```python
from build123d import *

# Parameters (mm, degrees)
F0_W     = 84
F0_H     = 80
F0_R     = 14
F0_R_2   = 16
F1_DEPTH = 225
F2_R     = 16
F2_R_2   = 14
F3_DEPTH = 100
F4_SIZE  = 1
F5_R     = 2.5
F6_DEPTH = 25
F7_R     = 2.5
F8_DEPTH = 25


# Not quite as in the source:
# - a feature names something its author has since deleted; it is built from what else it names


with BuildPart() as f1:
    # F0 (on Front) → F1 (new body)
    with BuildSketch(Plane.XZ):
        Rectangle(F0_W, F0_H)
        with Locations((-21, -19)):
            Circle(F0_R, mode=Mode.SUBTRACT)
        with Locations((21, -19)):
            Circle(F0_R_2, mode=Mode.SUBTRACT)
    extrude(amount=-F1_DEPTH)

    # F2 (on face) → F3 (cut)
    with BuildSketch(Plane(origin=(-42, 0, 0), x_dir=(0, -1, 0), z_dir=(-1, 0, 0))):
        with Locations((-204, 19)):
            Circle(F2_R)
        with Locations((-56, 19)):
            Circle(F2_R_2)
        with Locations((-21, 19)):
            Circle(F2_R)
    extrude(amount=-F3_DEPTH, mode=Mode.SUBTRACT)

    # F4
    f4_edges = [f1.edges().sort_by_distance(p)[0] for p in [
        (-42, 220, 19),
        (-42, 70, 19),
        (-42, 37, 19),
        (-35, 0, -19),
        (5, 0, -19),
        (42, 37, 19),
        (42, 70, 19),
        (42, 220, 19),
    ]]
    chamfer(f4_edges, length=F4_SIZE)

    # F5 (on face) → F6 (cut)
    with BuildSketch(Plane.XY.offset(40)):
        with Locations((21, 204)):
            Circle(F5_R)
        with Locations((21, 56)):
            Circle(F5_R)
        with Locations((21, 21)):
            Circle(F5_R)
        with Locations((-21, 21)):
            Circle(F5_R)
        with Locations((-21, 56)):
            Circle(F5_R)
        with Locations((-21, 204)):
            Circle(F5_R)
    extrude(amount=-F6_DEPTH, mode=Mode.SUBTRACT)

    # F7 (on face) → F8 (cut)
    with BuildSketch(Plane(origin=(0, 0, -40), x_dir=(1, 0, 0), z_dir=(0, 0, -1))):
        with Locations((-21, -21)):
            Circle(F7_R)
        with Locations((21, -21)):
            Circle(F7_R)
        with BuildLine():
            ThreePointArc((-18.5, -105), (-22.767766953, -103.232233047), (-21, -107.5))
            ThreePointArc((-21, -107.5), (-19.232233047, -106.767766953), (-18.5, -105))
        make_face()
        with BuildLine():
            ThreePointArc((-21, -152.5), (-22.767766953, -156.767766953), (-18.5, -155))
            ThreePointArc((-18.5, -155), (-19.232233047, -153.232233047), (-21, -152.5))
        make_face()
        with Locations((-21, -204)):
            Circle(F7_R)
        with Locations((21, -204)):
            Circle(F7_R)
    extrude(amount=-F8_DEPTH, mode=Mode.SUBTRACT)


solid = f1.part
```
Input: part model. Units: mm. Frame: model coordinates. A direction names the side the tool comes from. Coordinates: 2 decimals unless noted, no trailing zeros. Write each loop counter-clockwise with the first axis right and the second up, starting at its lowest first coordinate (ties: lowest second). Pieces come first, ordered by that corner, then holes.
1) Material intervals for line 1 along X through (y, z) = (56, 36); line 2 along Y through (x, z) = (-21, 38); line 3 along Y through (x, z) = (-21, -37), sorted ascending.
2) Mould query, pull axis Z, two halves, no side actions, for faces 1 (the flat face through (-1, 111, 40)), 2 (the cylindrical face through (-0.57, 24.47, 3.38)), 3 (the cylindrical face through (-0.574, 43.068, 13.638)), 4 (the cylindrical face through (-23.5, 20.9, -36.4)). Classes: pulls with the +Z half, pulls with the -Z half, needs draft (parallel to the pull), parting line crosses it, or undercut.
3) Section B-B on z = -19. Output: boundary loops of the cut face in (x, y), and give its area (3 significant figures).
4) Set-up query: faces 5 (the cylindrical face through (20.67, 206.48, 37.44)), 6 (the cylindrical face through (17.53, 111.43, -34.62)), 7 (the cylindrical face through (20.67, 201.52, -37.44)). Return all of +Z, -Z, +X, -X, +Y, -Y with unobstructed straight access to the full face (end or side cutting, diameter ignored); none if empty.
5) Section C-C on y = 204. Output: boundary loops of the cut face in (x, z).
6) Pin query (flat end, axial travel): pin 1 Ø3 at (x, y) = (-21, 204) entering from -Z; pin 2 Ø4 at (x, y) = (21, 204) entering from -Z. Return the tip coordinate at first contact, or that it passes through.
7) Section D-D on z = 19. Output: boundary loops of the cut face in (x, y), and give its area (3 significant figures).
8) Section A-A on x = 21. State how many separate pieces and enclosed holes the cut face has, and give its area (3 significant figures).
Check result:
1. line 1: x = -42 to -23.5, -18.5 to 18.5, 23.5 to 42
1. line 2: y = 0 to 18.5, 23.5 to 53.5, 58.5 to 201.5, 206.5 to 225
1. line 3: y = 0 to 18.5, 23.5 to 102.5, 107.5 to 152.5, 157.5 to 201.5, 206.5 to 225
2. face 1: pulls with the +Z half
2. face 2: undercut
2. face 3: undercut
2. face 4: needs draft
3. outline: (-42, 0) - (-36, 0) - (-35, 1) - (-35, 225) - (-42, 225) - close; (-7, 1) - (-6, 0) - (4, 0) - (5, 1) - (5, 225) - (-7, 225) - close; (37, 1) - (38, 0) - (42, 0) - (42, 225) - (37, 225) - close
3. area: 5,400 mm2
4. face 5: +Z
4. face 6: +Y, -Y
4. face 7: -Z
5. outline: (-42, -40) - (-23.5, -40) - (-23.5, -32.77) arc R14 cw (long way) to (-18.5, -32.77) - (-18.5, -40) - (18.5, -40) - (18.5, -34.8) arc R16 cw (long way) to (23.5, -34.8) - (23.5, -40) - (42, -40) - (42, 2) - (41, 3) - (-41, 3) - (-42, 2) - close; (-42, 36) - (-41, 35) - (-23.5, 35) - (-23.5, 40) - (-42, 40) - close; (-18.5, 35) - (18.5, 35) - (18.5, 40) - (-18.5, 40) - close; (23.5, 35) - (41, 35) - (42, 36) - (42, 40) - (23.5, 40) - close
6. pin 1: stops at z = -5.08
6. pin 2: stops at z = -3.13
7. outline: (-42, 0) - (42, 0) - (42, 4) - (41, 5) - (-41, 5) - (-42, 4) - close; (-42, 38) - (-41, 37) - (41, 37) - (42, 38) - (42, 41) - (41, 42) - (-41, 42) - (-42, 41) - close; (-42, 71) - (-41, 70) - (41, 70) - (42, 71) - (42, 187) - (41, 188) - (-41, 188) - (-42, 187) - close; (-42, 221) - (-41, 220) - (41, 220) - (42, 221) - (42, 225) - (-42, 225) - close
7. area: 11,200 mm2
8. separate pieces: 4
8. enclosed holes: 0
8. area: 8,440 mm2
